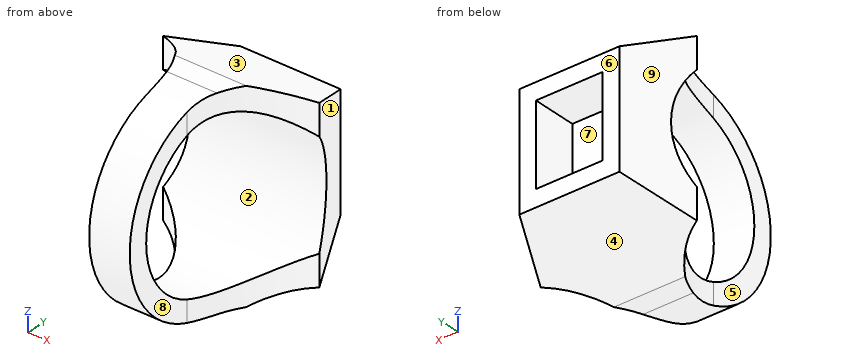
```python
from build123d import *

# Parameters (mm, degrees)
SKETCH_1_R                    = 12
EXTRUDE_1_DEPTH               = 25
CUT_EXTRUDE_1_DEPTH           = 35.263683398
CUT_EXTRUDE_1_DEPTH_BACK      = 35.263683398
SKETCH_2_OUTSIDE_W            = 65.4
SKETCH_2_OUTSIDE_H            = 48.4
SKETCH_3_W                    = 10
SKETCH_3_H                    = 12
CUT_EXTRUDE_2_DEPTH           = 5
CUT_EXTRUDE_2_TAPER           = 15
CUT_EXTRUDE_2_OTHER_WAY_DEPTH = 39.089557823


with BuildPart() as part:
    # 草图1 → 凸台-拉伸1 (new, symmetric)
    with BuildSketch(Plane(origin=(0, 0, 0), x_dir=(0, 0, -1), z_dir=(1, 0, 0))):
        with BuildLine():
            Line((-8.5, 18), (8.5, 18))
            Line((8.5, 18), (15, 3.40076097))
            Line((15, 3.40076097), (15, 0))
            ThreePointArc((15, 0), (0, -15), (-15, 0))
            Line((-15, 0), (-15, 3.40076097))
            Line((-15, 3.40076097), (-8.5, 18))
        make_face()
        Circle(SKETCH_1_R, mode=Mode.SUBTRACT)
    extrude(amount=EXTRUDE_1_DEPTH, both=True)

    # 草图2 outside → 切除-拉伸1 (cut, two sides: drawn at the far end of the back side and taken through both)
    with BuildSketch(Plane.XY.offset(-CUT_EXTRUDE_1_DEPTH_BACK)):
        with Locations((0, 1.5)):
            Rectangle(SKETCH_2_OUTSIDE_W, SKETCH_2_OUTSIDE_H)
        with BuildLine():
            Line((-7.5, 18), (7.5, 18))
            Line((7.5, 18), (11.696768923, 9))
            ThreePointArc((11.696768923, 9), (5.385171162, 3.46487732), (3.03604285, -4.594616806))
            Line((3.03604285, -4.594616806), (3.03604285, -15))
            Line((3.03604285, -15), (-3.03604285, -15))
            Line((-3.03604285, -15), (-3.03604285, -4.594616806))
            ThreePointArc((-3.03604285, -4.594616806), (-5.385171162, 3.46487732), (-11.696768923, 9))
            Line((-11.696768923, 9), (-7.5, 18))
        make_face(mode=Mode.SUBTRACT)
    extrude(amount=CUT_EXTRUDE_1_DEPTH + CUT_EXTRUDE_1_DEPTH_BACK, mode=Mode.SUBTRACT)

    # 草图3 → 切除-拉伸2 (cut)
    with BuildSketch(Plane(origin=(0, 18, 0), x_dir=(1, 0, 0), z_dir=(0, 1, 0))):
        Rectangle(SKETCH_3_W, SKETCH_3_H)
    extrude(amount=-CUT_EXTRUDE_2_DEPTH, taper=CUT_EXTRUDE_2_TAPER, mode=Mode.SUBTRACT)

    # 草图3 → 切除-拉伸2 other way (cut)
    with BuildSketch(Plane(origin=(0, 18, 0), x_dir=(1, 0, 0), z_dir=(0, 1, 0))):
        Rectangle(SKETCH_3_W, SKETCH_3_H)
    extrude(amount=CUT_EXTRUDE_2_OTHER_WAY_DEPTH, mode=Mode.SUBTRACT)


solid = part.part
```
Source: CAD feature listing. Evaluate the final solid. Frame: model axes, mm. Face numbers are marked on the shaded views. A direction names the side the tool comes from. Coordinates: 2 decimals unless noted, no trailing zeros. Order: outer loops, then holes, each group sorted by start corner. A loop starts at its lowest first (then second) coordinate and runs counter-clockwise, first axis right, second up. Notation, with made-up numbers: M 72,-8 L 103,-8 A29 ccw 103,27 Z; hole C -33.75,-18 d2. An arc over 180 degrees is marked long. Write each question's results on one line, items separated by ' | '. Start each with the question number.
1) Section query A-A (y = -8.5). Return the cut outline in (x, z).
2) Contact query for flat-ended pins moving along their axis: pin 1 Ø5 at (x, z) = (1, 9.5) entering from -Y; pin 2 Ø3 at (y, z) = (-11.5, -3) entering from -X; pin 3 Ø2 at (x, z) = (0.5, -0.5) entering from +Y; pin 4 Ø3 at (y, z) = (-9.5, 3.5) entering from +X. Output: stop coordinate, or through.
3) Section query B-B (y = 1). Return the cut outline in (x, z), plus the area to 3 significant figures.
4) Section query C-C (x = -9). Return the cut outline in (y, z).
5) Draft query along Z for the marked faces 1, 2, 3 and 4. Return one class per face: released by +Z, released by -Z, zero draft, split by the parting line, or undercut.
6) Line query: line 1 (Y direction, x = -0.5, z = 0); line 2 (Z direction, x = -1.5, y = 0); line 3 (Y direction, x = 7, z = 0). Output: solid intervals per line, ascending. Write a range as from..to.
7) Access query for the marked faces 5, 6, 7, 8 and 9. Directions: +Z, -Z, +X, -X, +Y, -Y. A direction counts if a zero-diameter tool reaches every point of the face in a straight line with its end or side. Return the directions, or none.
Answers:
1) outline: M -3.04,-12.36 L 3.04,-12.36 L 3.04,-8.47 L -3.04,-8.47 Z; M -3.04,8.47 L 3.04,8.47 L 3.04,12.36 L -3.04,12.36 Z
2) pin 1: stops at y = -13.27 | pin 2: stops at x = -3.04 | pin 3: stops at y = 13 | pin 4: passes through
3) outline: M -4.12,-15 L 4.12,-15 L 4.12,-11.96 L -4.12,-11.96 Z; M -4.12,11.96 L 4.12,11.96 L 4.12,15 L -4.12,15 Z | area: 50.1 mm^2
4) outline: M 7.38,-13.23 L 14.78,-9.93 L 14.78,9.93 L 7.38,13.23 L 7.38,9.46 A12 cw 7.38,-9.46 Z
5) face 1: zero draft | face 2: undercut | face 3: released by +Z | face 4: released by -Z
6) line 1: y = -15..-12, 12..13 | line 2: z = -15..-12, 12..15 | line 3: y = 12..18
7) face 5: +Z, -Z, -X, -Y | face 6: +Z, -Z, +X, -X, +Y | face 7: +Y | face 8: +Z, -Z, +X, -Y | face 9: +Z, -Z, -X, +Y
